Input: part model. Units: mm. Frame: model coordinates. A direction names the side the tool comes from. Round coordinates to 2 decimals unless told otherwise and drop trailing zeros. Write each loop counter-clockwise with the first axis right and the second up, starting at its lowest first coordinate (ties: lowest second). Pieces come first, ordered by that corner, then holes. Notation, with made-up numbers: (7.5, 61) - (53.5, 61) arc R23 ccw to (53.5, 76) - close; hole circle Ø5 at (70, 18). An arc over 180 degrees is marked (long way). Use one line per item in the form item = value.
```python
from build123d import *

# Parameters (mm, degrees)
F0_W     = 77.468356
F0_H     = 26.487343
F1_DEPTH = 25
F2_W     = 69.778483
F2_H     = 19.08228
F3_DEPTH = 23
F4_W     = 3
F4_H     = 23
F5_DEPTH = 10
F6_R     = 3.973158
F7_DEPTH = 72


with BuildPart() as f1:
    # F0 (on Top) → F1 (new body)
    with BuildSketch(Plane.XY):
        with Locations((16.091772, 5.268987)):
            Rectangle(F0_W, F0_H)
    extrude(amount=F1_DEPTH)

    # F2 (on Top) → F3 (cut)
    with BuildSketch(Plane.XY):
        with Locations((15.949367, 4.984178)):
            Rectangle(F2_W, F2_H)
    extrude(amount=F3_DEPTH, mode=Mode.SUBTRACT)

    # F4 (on Front) → F5 (join)
    with BuildSketch(Plane.XZ):
        with Locations((-21.174206, -8.476495)):
            Rectangle(F4_W, F4_H)
        with Locations((52.004144, -11.5)):
            Rectangle(F4_W, F4_H)
    extrude(amount=-F5_DEPTH)

    # F6 (on face) → F7 (join)
    with BuildSketch(Plane.YZ.offset(-19.674206)):
        with Locations((4.750193, -14.371534)):
            Circle(F6_R)
    extrude(amount=F7_DEPTH)


solid = f1.part
```
(1) Access query for faces 1 (the face through (53.504, 5, -12)), 2 (the face through (16, 18.513, 12)), 3 (the face through (52, 0, -11)), 4 (the face through (15, 14.525, 11)), 5 (the face through (50.839, 5, 11)). Directions: +Z, -Z, +X, -X, +Y, -Y. A direction counts if a zero-diameter tool reaches every point of the face in a straight line with its end or side. Return the directions, or none.
Derived:
face_1 = -Z, +X, +Y, -Y
face_2 = +Z, -Z, +X, -X, +Y
face_3 = -Z, +X, -X, -Y
face_4 = -Z
face_5 = none
(2) Cut plane A-A on z = 8.5. Output: boundary loops of the cut face in (x, y).
Derived:
outline = (-22.64, -7.97) - (54.83, -7.97) - (54.83, 18.51) - (-22.64, 18.51) - close; hole (-18.94, -4.56) - (50.84, -4.56) - (50.84, 14.53) - (-18.94, 14.53) - close
(3) Draft query along Z for faces 6 (the face through (14.92, 3.89, -18.25)), 7 (the face through (54.826, 5, 12)), 8 (the face through (-21, 5, -19.976)). Return one class per face: released by +Z, released by -Z, zero draft, split by the parting line, or undercut.
Derived:
face_6 = undercut
face_7 = zero draft
face_8 = released by -Z
(4) Material intervals for L1, parallel to Y at x = -13, z = 14.5; L2, parallel to X at y = 0.5, z = 13; L3, parallel to X at y = 8, z = 0.5, sorted ascending.
Derived:
L1 = -7.97 to -4.56, 14.53 to 18.51
L2 = -22.64 to -18.94, 50.84 to 54.83
L3 = -22.67 to -18.94, 50.84 to 54.83
(5) Cut plane D-D on y = -2.25. Output: boundary loops of the cut face in (x, z), then the cut area to 3 significant figures.
Derived:
outline = (-22.64, 0) - (-18.94, 0) - (-18.94, 23) - (50.84, 23) - (50.84, 0) - (54.83, 0) - (54.83, 25) - (-22.64, 25) - close
area = 332 mm^2
(6) Cut plane C-C on x = -14. Output: boundary loops of the cut face in (y, z).
Derived:
outline = (-7.97, 0) - (-4.56, 0) - (-4.56, 23) - (14.53, 23) - (14.53, 0) - (18.51, 0) - (18.51, 25) - (-7.97, 25) - close; circle Ø7.95 at (4.75, -14.37)
(7) Cut plane B-B on z = -3. Output: boundary loops of the cut face in (x, y).
Derived:
outline = (-22.67, 0) - (-19.67, 0) - (-19.67, 10) - (-22.67, 10) - close; (50.5, 0) - (53.5, 0) - (53.5, 10) - (50.5, 10) - close
(8) First-contact query: pin 1 Ø2 at (x, y) = (10.5, 14) entering from -Z; pin 2 Ø0.9 at (x, z) = (-21.5, -3.5) entering from -Y; pin 3 Ø9.5 at (x, y) = (6.5, 1.5) entering from -Z; pin 4 Ø3 at (x, z) = (30.5, -7.5) entering from +Y. Flat tips, straight axial feed; report the tip coordinate or a pass-through.
Derived:
pin_1 = 0
pin_2 = 0
pin_3 = -18.34
pin_4 = through
